```python
from build123d import *

# Parameters (mm, degrees)
F0_W      = 457.2
F0_H      = 203.2
F1_DEPTH  = 12.7
F2_W      = 127
F2_H      = 190.5
F3_DEPTH  = 9.525
F5_D      = 11.1125
F7_DEPTH  = 4.7625
F9_DEPTH  = 4.7625
F10_W     = 25.4
F10_H     = 454.152
F11_DEPTH = 101.6
F12_W     = 44.551104
F12_H     = 159.36184
F13_DEPTH = 203.201
F14_W     = 96.83972
F14_H     = 38.1
F15_DEPTH = 203.201
F17_D     = 17.4625


with BuildPart() as f1:
    # F0 (on Top) → F1 (new body)
    with BuildSketch(Plane.XY):
        Rectangle(F0_W, F0_H)
    extrude(amount=F1_DEPTH)

    # F2 (on face) → F3 (join)
    with BuildSketch(Plane.XY.offset(12.7)):
        with Locations((158.75, 0)):
            Rectangle(F2_W, F2_H)
        with Locations((-158.75, 0)):
            Rectangle(F2_W, F2_H)
    extrude(amount=F3_DEPTH)

    # F5 (through all)
    with Locations(Plane.XY.offset(22.225)):
        with Locations((-196.85, 61.976), (-120.65, 61.976), (-196.85, -61.976), (-120.65, -61.976), (120.65, 61.976), (196.85, 61.976), (196.85, -61.976), (120.65, -61.976)):
            Hole(F5_D / 2)

    # F6 (on Front) → F7 (join, symmetric)
    with BuildSketch(Plane.XZ):
        Polygon((-95.25, 0), (-222.25, 0), (-222.25, -25.4), (-120.65, -127), (-95.25, -127), align=None)
    extrude(amount=F7_DEPTH, both=True)

    # F8 (on Front) → F9 (join, symmetric)
    with BuildSketch(Plane.XZ):
        Polygon((222.25, -25.4), (222.25, 0), (-69.85, 0), (-69.85, -454.152), (-44.45, -454.152), align=None)
    extrude(amount=F9_DEPTH, both=True)

    # F10 (on Front) → F11 (join, symmetric)
    with BuildSketch(Plane.XZ):
        with Locations((-82.55, -227.076)):
            Rectangle(F10_W, F10_H)
    extrude(amount=F11_DEPTH, both=True)

    # F12 (on face) → F13 (cut, through all)
    with BuildSketch(Plane.XZ.offset(101.6)):
        with Locations((-111.175552, -381.43292)):
            Rectangle(F12_W, F12_H)
    extrude(amount=-F13_DEPTH, mode=Mode.SUBTRACT)

    # F14 (on face) → F15 (cut, through all)
    with BuildSketch(Plane.XZ.offset(101.6)):
        with Locations((-130.46186, -384.175)):
            Rectangle(F14_W, F14_H)
    extrude(amount=-F15_DEPTH, mode=Mode.SUBTRACT)

    # F17 (through all)
    with Locations(Plane.YZ.offset(-69.85)):
        with Locations((-82.55, -346.075), (-82.55, -422.275), (82.55, -422.275), (82.55, -346.075)):
            Hole(F17_D / 2)


solid = f1.part
```
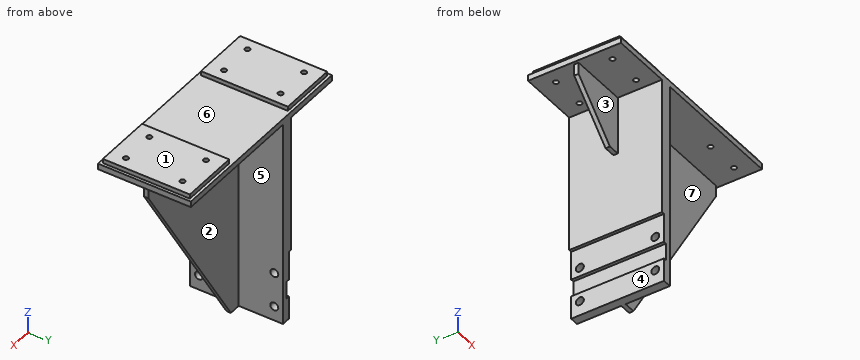
Here's how the part is built. I have some questions about the finished solid (model axes, mm). Face numbers are marked on the shaded views. A direction names the side the tool comes from. Round coordinates to 2 decimals unless told otherwise and drop trailing zeros. Loops run counter-clockwise (first coordinate to the right, second up) from the corner with the lowest first, then second, coordinate; pieces in that order, holes last.
1. For the marked faces 1, 2, 3 and 4, which set-ups out of +Z, -Z, +X, -X, +Y, -Y let a thin tool reach every point of the face, with its end or its side?
Answers:
face 1: +Z, +X, -X, +Y, -Y
face 2: -Z, +X, +Y
face 3: -Z, -X, -Y
face 4: -Z, -X, +Y, -Y
2. Suppose I cut it at A-A, the plane y = -82.55. Give the number of separate pieces and of enclosed holes in the cut face, and give its area (3 significant figures).
Answers:
separate pieces: 3
enclosed holes: 0
area: 17,900 mm2
3. Will these pins go through, and if not, where does the flat tip stop? pin 1 (20 mm diameter, centred on y = 82.55, z = -346.075, fed in from -X); pin 2 (5 mm diameter, centred on x = 131.5, y = -58.5, fed in from -Z); pin 3 (1.5 mm diameter, centred on y = 37, z = -207.5, fed in from +X).
Answers:
pin 1: stops at x = -88.9
pin 2: stops at z = 0
pin 3: stops at x = -69.85
4. If I drill on probe 1 along Y at (x, z) = (-196, 11); probe 2 along Z at (x, y) = (-76, 82.55); probe 3 along Y at (x, z) = (-196.85, 14), over which ranges is the centre line in solid material (lowest first)?
Answers:
probe 1: y = -101.6 to -67.47, -56.49 to 56.49, 67.47 to 101.6
probe 2: z = -454.15 to -431.01, -413.54 to -354.81, -337.34 to 12.7
probe 3: y = -95.25 to -67.53, -56.42 to 56.42, 67.53 to 95.25
5. Suppose I cut it at C-C, the plane z = -7. Please give me the cut outline in (x, y).
Answers:
outline: (-222.25, -4.76) - (-95.25, -4.76) - (-95.25, -101.6) - (-69.85, -101.6) - (-69.85, -4.76) - (222.25, -4.76) - (222.25, 4.76) - (-69.85, 4.76) - (-69.85, 101.6) - (-95.25, 101.6) - (-95.25, 4.76) - (-222.25, 4.76) - close
6. Thinking about a two-plate mould opening in X: for the marked faces 5, 6 and 7, which applies, released by +X, released by -X, zero draft, split by the parting line, or undercut?
Answers:
face 5: released by +X
face 6: undercut
face 7: zero draft
